Here's how the part is built. I have some questions about the finished solid (model axes, mm). Coordinates: 2 decimals unless noted, no trailing zeros. Order: outer loops, then holes, each group sorted by start corner. A loop starts at its lowest first (then second) coordinate and runs counter-clockwise, first axis right, second up. Notation, with made-up numbers: (-2, -34.75) - (50, -34.75) arc R24 cw to (50, -12.75) - close; hole circle Ø9 at (-9, 58.25). An arc over 180 degrees is marked (long way). Answer in a Markdown table with one row per item. Add a question column.
Item 1: Will these pins go through, and if not, where does the flat tip stop? pin 1 Ø2.5 at (x, z) = (0, 0) entering from -Y; pin 2 Ø6.5 at (x, z) = (0, 0) entering from +Y.
Item 2: If I drill on line 1 along X through (y, z) = (10, 0), over which ranges is the centre line in solid material (lowest first)? Write a range as from..to.
Item 3: I want a section at A-A (z = 0). Please give me the cut outline in (x, y).
Item 4: I want a section at B-B (x = 0). Please give me the cut outline in (y, z).
```python
from build123d import *

# Parameters (mm, degrees)
CROQUIS_BASE_W             = 75
CROQUIS_BASE_H             = 75
COLUMNA_75X150_DEPTH       = 150
CROQUIS_AGUJEROS_MONTAJE_R = 4
AGUJERO_INSERTO_M6_DEPTH   = 14
AGUJERO_SUPERIOR_M6_START  = -14
CROQUIS_AGUJERO_SUPERIOR_R = 4
AGUJERO_SUPERIOR_M6_DEPTH  = 14


with BuildPart() as part:
    # Croquis_base → Columna_75x150 (new body)
    with BuildSketch(Plane(origin=(0, 0, 0), x_dir=(1, 0, 0), z_dir=(0, 1, 0))):
        Rectangle(CROQUIS_BASE_W, CROQUIS_BASE_H)
    extrude(amount=COLUMNA_75X150_DEPTH)

    # Croquis_agujeros_montaje → Agujero_inserto_M6 (cut)
    with BuildSketch(Plane(origin=(0, 0, 0), x_dir=(1, 0, 0), z_dir=(0, 1, 0))):
        with Locations(Location((0, 0, 0), (0, 0, 270))):
            Circle(CROQUIS_AGUJEROS_MONTAJE_R)
    extrude(amount=AGUJERO_INSERTO_M6_DEPTH, mode=Mode.SUBTRACT)

    # Croquis_agujero_superior → Agujero_superior_M6 (cut)
    with BuildSketch(Plane(origin=(0, 150, 0), x_dir=(1, 0, 0), z_dir=(0, 1, 0)).offset(AGUJERO_SUPERIOR_M6_START)):
        with Locations(Location((0, 0, 0), (0, 0, 270))):
            Circle(CROQUIS_AGUJERO_SUPERIOR_R)
    extrude(amount=AGUJERO_SUPERIOR_M6_DEPTH, mode=Mode.SUBTRACT)


solid = part.part
```
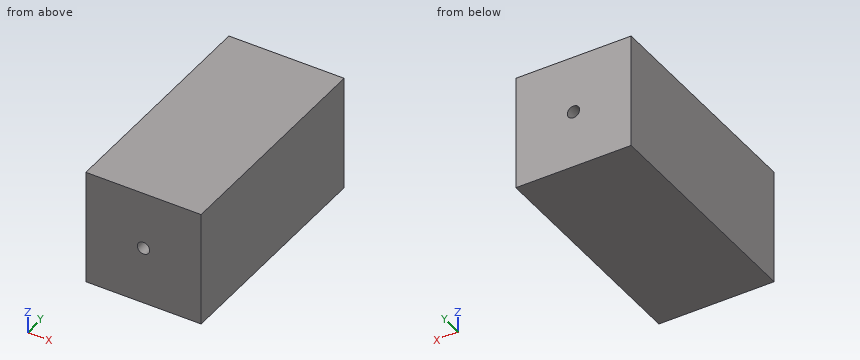
Values follow:
| question | item | result |
|---|---|---|
| 1 | pin 1 | stops at y = 14 |
| 1 | pin 2 | stops at y = 136 |
| 2 | line 1 | x = -37.5..-4, 4..37.5 |
| 3 | outline | (-37.5, 0) - (-4, 0) - (-4, 14) - (4, 14) - (4, 0) - (37.5, 0) - (37.5, 150) - (4, 150) - (4, 136) - (-4, 136) - (-4, 150) - (-37.5, 150) - close |
| 4 | outline | (0, -37.5) - (150, -37.5) - (150, -4) - (136, -4) - (136, 4) - (150, 4) - (150, 37.5) - (0, 37.5) - (0, 4) - (14, 4) - (14, -4) - (0, -4) - close |
